Geometry check sheet. Reference: the model listing, model coordinates, mm. A direction names the side the tool comes from. Coordinates: 2 decimals unless noted, no trailing zeros. Write each loop counter-clockwise with the first axis right and the second up, starting at its lowest first coordinate (ties: lowest second). Pieces come first, ordered by that corner, then holes. Notation, with made-up numbers: M 75.25,-9.75 L 102.25,-9.75 A25 ccw 102.25,20.25 Z; hole C 54.5,37.5 d3. An arc over 180 degrees is marked long. Put each result on its own line as item: value. Start each with the question number.
1) Set-up check for faces 1 (the flat face through (88, -11.556, 3)), 2 (the cylindrical face through (38.49, 4.28, 2.96)), 3 (the flat face through (-5, -51.556, 3)): record each of +Z, -Z, +X, -X, +Y, -Y from which the full face is reachable in a straight line by a thin tool's end or side.
2) Cross-section at B-B on y = -15. Record the cut outline in (x, z).
3) Scan lines: line 1 along Y through (x, z) = (72, 4.9); line 2 along X through (y, z) = (-17.5, 1.35); line 3 along Y through (x, z) = (-26, 4.1). Record each from-to range of solid material in increasing order.
4) Gauge pin test, flat ends, axial feed: pin 1 (3.5 mm diameter, centred on y = 50.5, z = 4.5, fed in from +X); pin 2 (1.8 mm diameter, centred on y = -55, z = 1.5, fed in from +X); pin 3 (1.8 mm diameter, centred on y = -55, z = 2.5, fed in from -X). Record the tip position at first contact, or that the pin passes through.
5) Cross-section at A-A on x = -72.5. Record the cut outline in (y, z).
6) Mould release check, pull along Y, two halves, no side actions. Record for faces 4 (the flat face through (-98, 28.444, 3)), 5 (the flat face through (24.645, -55, 3)), 6 (the flat face through (78, 5.444, 3)): released by +Y, released by -Y, zero draft, split by the parting line, or undercut.
from build123d import *

# Parameters (mm, degrees)
SKETCH1_R           = 4
BOSS_EXTRUDE1_DEPTH = 6


with BuildPart() as part:
    # Sketch1 → Boss-Extrude1 (new body)
    with BuildSketch(Plane.XY):
        with BuildLine():
            Line((-95.354884471, 28.444147702), (-95.354884471, 8.444147702))
            Line((-95.354884471, 8.444147702), (-101.354884471, 8.444147702))
            Line((-101.354884471, 8.444147702), (-101.354884471, -11.555852298))
            Line((-101.354884471, -11.555852298), (-95.354884471, -11.555852298))
            Line((-95.354884471, -11.555852298), (-95.354884471, -31.555852298))
            Line((-95.354884471, -31.555852298), (-101.354884471, -31.555852298))
            Line((-101.354884471, -31.555852298), (-101.354884471, -51.555852298))
            Line((-101.354884471, -51.555852298), (-75.354884471, -51.555852298))
            Line((-75.354884471, -51.555852298), (-75.354884471, -57.555852298))
            Line((-75.354884471, -57.555852298), (-55.354884471, -57.555852298))
            Line((-55.354884471, -57.555852298), (-55.354884471, -51.555852298))
            Line((-55.354884471, -51.555852298), (-35.354884471, -51.555852298))
            Line((-35.354884471, -51.555852298), (-35.354884471, -57.555852298))
            Line((-35.354884471, -57.555852298), (-15.354884471, -57.555852298))
            Line((-15.354884471, -57.555852298), (-15.354884471, -51.555852298))
            Line((-15.354884471, -51.555852298), (4.645115529, -51.555852298))
            Line((4.645115529, -51.555852298), (4.645115529, -57.555852298))
            Line((4.645115529, -57.555852298), (24.645115529, -57.555852298))
            Line((24.645115529, -57.555852298), (24.645115529, -51.555852298))
            Line((24.645115529, -51.555852298), (44.645115529, -51.555852298))
            Line((44.645115529, -51.555852298), (44.645115529, -57.555852298))
            Line((44.645115529, -57.555852298), (64.645115529, -57.555852298))
            Line((64.645115529, -57.555852298), (64.645115529, -51.555852298))
            Line((64.645115529, -51.555852298), (90.645115529, -51.555852298))
            Line((90.645115529, -51.555852298), (90.645115529, -31.555852298))
            Line((90.645115529, -31.555852298), (84.645115529, -31.555852298))
            Line((84.645115529, -31.555852298), (84.645115529, -11.555852298))
            Line((84.645115529, -11.555852298), (90.645115529, -11.555852298))
            Line((90.645115529, -11.555852298), (90.645115529, 5.444147702))
            Line((90.645115529, 5.444147702), (64.645115529, 5.444147702))
            Line((64.645115529, 5.444147702), (64.645115529, 2.444147702))
            Line((64.645115529, 2.444147702), (47.89113696, 2.444147702))
            ThreePointArc((47.89113696, 2.444147702), (38.36080563, 4.331969424), (30.269799621, 9.710324922))
            Line((30.269799621, 9.710324922), (-1.398719, 41.177970481))
            ThreePointArc((-1.398719, 41.177970481), (-9.48972501, 46.55632598), (-19.020056339, 48.444147702))
            Line((-19.020056339, 48.444147702), (-35.354884471, 48.444147702))
            Line((-35.354884471, 48.444147702), (-35.354884471, 51.444147702))
            Line((-35.354884471, 51.444147702), (-55.354884471, 51.444147702))
            Line((-55.354884471, 51.444147702), (-55.354884471, 48.444147702))
            Line((-55.354884471, 48.444147702), (-75.354884471, 48.444147702))
            Line((-75.354884471, 48.444147702), (-75.354884471, 51.444147702))
            Line((-75.354884471, 51.444147702), (-101.354884471, 51.444147702))
            Line((-101.354884471, 51.444147702), (-101.354884471, 28.444147702))
            Line((-101.354884471, 28.444147702), (-95.354884471, 28.444147702))
        make_face()
        with Locations((-65.354884471, -40.555852298)):
            Circle(SKETCH1_R, mode=Mode.SUBTRACT)
    extrude(amount=BOSS_EXTRUDE1_DEPTH)


solid = part.part
Answer key:
1. face 1: +Z, -Z, +X
1. face 2: +Z, -Z, +Y
1. face 3: +Z, -Z, -Y
2. outline: M -95.35,0 L 84.65,0 L 84.65,6 L -95.35,6 Z
3. line 1: y = -51.56 to 5.44
3. line 2: x = -95.35 to 84.65
3. line 3: y = -57.56 to 48.44
4. pin 1: stops at x = -35.35
4. pin 2: stops at x = 64.65
4. pin 3: stops at x = -75.35
5. outline: M -57.56,0 L 48.44,0 L 48.44,6 L -57.56,6 Z
6. face 4: undercut
6. face 5: zero draft
6. face 6: released by +Y
